Input: part model. Units: mm. Frame: model coordinates. Face numbers are marked on the shaded views. Coordinates: 2 decimals unless noted, no trailing zeros. Use a Markdown table: item, result. Add a question column.
1. Draft query along X for the marked faces 1, 2 and 3. Return one class per face: released by +X, released by -X, zero draft, split by the parting line, or undercut.
2. Contact query for flat-ended pins moving along their axis: P1, Ø8, axis at x = 10, y = 5, coming from the +Z side; P2, Ø10, axis at x = 36, y = -17.5, coming from the -Z side; P3, Ø16, axis at x = -13, y = 23, coming from the -Z side. Output: stop coordinate, or through.
3. Ray query, L1, parallel to X at y = -9, z = 14.5 (3 decimals); L2, parallel to Y at x = -39.6, z = 0 (3 decimals); L3, parallel to Y at x = -5, z = 0 (3 decimals). Return the intervals inside material, ascending. Write a range as [from, to].
4. Section query A-A on z = 17.5. State how many separate pieces and enclosed holes the cut face has, then the cut area to 3 significant figures.
```python
from build123d import *

# Parameters (mm, degrees)
F3_DEPTH = 1.5875
F4_COUNT = 4
F5_R     = 9.525
F5_R_2   = 6.35
F6_DEPTH = 22.225


with BuildPart() as f1:
    # F0 (on Front) → F1 (revolve)
    with BuildSketch(Plane.XZ):
        with BuildLine():
            Line((-6.35, 21.5449612588), (0, 21.5449612588))
            add(Edge.make_bspline(
                [(0, 21.5449612588), (5.7091140074, 17.8062328478), (14.9433568334, 11.7590027587), (22.6094264222, 12.0531771122), (41.7193795404, 20.2005543654), (55.0581365824, 25.8874278516)],
                knots=[0, 0, 0, 0, 0.3284545806, 0.5312609541, 1, 1, 1, 1], degree=3))
            Line((55.0581365824, 25.8874278516), (54.1192181408, 28.3520705998))
            add(Edge.make_bspline(
                [(0, 24.0849612588), (5.828247379, 20.394150502), (15.2551832359, 14.4244251281), (21.3280668754, 14.1649541634), (50.7778755781, 26.425568968), (53.4362491864, 27.9582945111), (54.1192181408, 28.3520705998)],
                knots=[0, 0, 0, 0, 0.2932614007, 0.474337521, 0.8649508284, 1, 1, 1, 1], degree=3))
            Line((0, 24.0849612588), (0, 28.575))
            Line((0, 28.575), (-6.35, 28.575))
            Line((-6.35, 28.575), (-6.35, 21.5449612588))
        make_face()
    revolve(axis=Axis((-21.6108541936, 0, 0), (-1, 0, 0)))



with BuildPart() as f1b:
    # F0 (on Front) → F1, piece 2 (revolve)
    with BuildSketch(Plane.XZ):
        with BuildLine():
            Line((-25.4, 13.961916452), (-25.4, 19.05))
            Line((-25.4, 19.05), (-28.575, 19.05))
            Line((-28.575, 19.05), (-28.575, 15.1060059758))
            Line((-28.575, 15.1060059758), (-39.4406318665, 19.0213620663))
            Line((-39.4406318665, 19.0213620663), (-47.7628409863, 19.0213620663))
            Line((-47.7628409863, 19.0213620663), (-47.7628409863, 12.7))
            Line((-47.7628409863, 12.7), (-55.2181527019, 12.7))
            Line((-55.2181527019, 12.7), (-55.2181527019, 22.7018314168))
            Line((-55.2181527019, 22.7018314168), (-61.9799494743, 22.7018314168))
            Line((-61.9799494743, 22.7018314168), (-61.9799494743, 12.7))
            Line((-61.9799494743, 12.7), (-61.9799494743, 9.525))
            Line((-61.9799494743, 9.525), (-39.4406318665, 9.525))
            add(Edge.make_bspline(
                [(-39.4406318665, 9.525), (-35.4392920306, 9.9052529375), (-26.9580608884, 10.71123623), (-17.8813827929, 6.392138264), (-13.0869690329, 4.1107372381)],
                knots=[0, 0, 0, 0, 0.4717876177, 1, 1, 1, 1], degree=3))
            Line((-13.0869690329, 4.1107372381), (-13.0869690329, 9.525))
            Line((-13.0869690329, 9.525), (-25.4, 13.961916452))
        make_face()
    revolve(axis=Axis((-21.6108541936, 0, 0), (-1, 0, 0)))


with BuildPart() as f1_1:
    add(f1.part)

    add(f1b.part)  # F3 merges F1b
    # F2 (on Front) → F3 (join, symmetric)
    with BuildSketch(Plane.XZ):
        Polygon((-6.2443618663, 28.5232551396), (-25.5005825311, 18.9564712346), (-25.5005825311, 14.0504268929), (-6.3670128584, 18.9564712346), align=None)
    extrude(amount=F3_DEPTH, both=True)

    # F4: F1 ×4 about axis
    f4_axis = Axis((-21.6108541936, 0, 0), (-1, 0, 0))


with BuildPart() as f1_2:
    add(f1_1.part)
    for i in range(1, F4_COUNT):
        add(f1_1.part.rotate(f4_axis, i * 360 / F4_COUNT))

    # F5 (on face) → F6 (join)
    with BuildSketch(Plane(origin=(-61.9799494743, 0, 0), x_dir=(0, -1, 0), z_dir=(-1, 0, 0))):
        Circle(F5_R)
        Circle(F5_R_2, mode=Mode.SUBTRACT)
    extrude(amount=-F6_DEPTH)


solid = f1_2.part
```
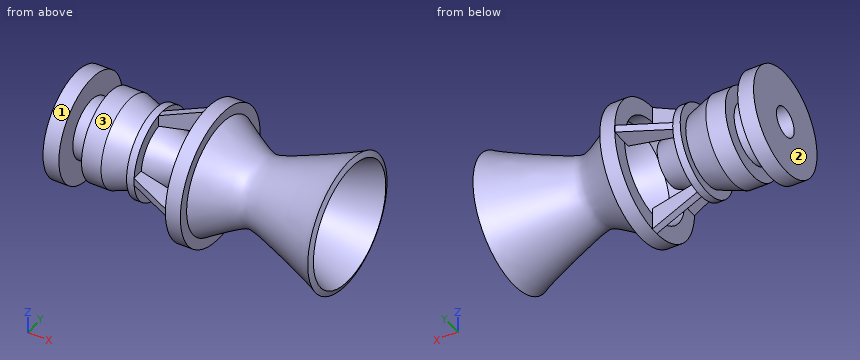
Resolved:
| question | item | result |
|---|---|---|
| 1 | face 1 | zero draft |
| 1 | face 2 | released by -X |
| 1 | face 3 | undercut |
| 2 | P1 | z = 19.84 |
| 2 | P2 | z = -16.92 |
| 2 | P3 | z = -21.73 |
| 3 | L1 | [-61.98, -55.218], [-47.763, -34.014], [-28.575, -25.4], [6.957, 11.498], [27.267, 33.975] |
| 3 | L2 | [-19.021, -9.525], [9.525, 19.021] |
| 3 | L3 | [-28.575, -21.545], [21.545, 28.575] |
| 4 | separate pieces | 5 |
| 4 | enclosed holes | 0 |
| 4 | area | 960 mm² |
